from build123d import *

# Parameters (mm, degrees)
SKETCH1_W           = 20
SKETCH1_H           = 46
SKETCH1_R           = 1.25
SKETCH1_R_2         = 4
SKETCH1_R_3         = 1.5
BOSS_EXTRUDE1_DEPTH = 3
SKETCH2_W           = 20
SKETCH2_H           = 13.653393661
CUT_EXTRUDE4_DEPTH  = 26.258661881


with BuildPart() as part:
    # Sketch1 → Boss-Extrude1 (new body)
    with BuildSketch(Plane(origin=(0, 0, 0), x_dir=(1, 0, 0), z_dir=(0, 1, 0))):
        Rectangle(SKETCH1_W, SKETCH1_H)
        with Locations(Location((0, 18, 0), (0, 0, 270))):
            Circle(SKETCH1_R, mode=Mode.SUBTRACT)
        with Locations(Location((0, 1, 0), (0, 0, 270))):
            Circle(SKETCH1_R, mode=Mode.SUBTRACT)
        with Locations(Location((0, 9.5, 0), (0, 0, 270))):
            Circle(SKETCH1_R_2, mode=Mode.SUBTRACT)
        with Locations(Location((0, -13, 0), (0, 0, 270))):
            Circle(SKETCH1_R_3, mode=Mode.SUBTRACT)
    extrude(amount=BOSS_EXTRUDE1_DEPTH)

    # Sketch2 → Cut-Extrude4 (cut, through all)
    with BuildSketch(Plane(origin=(0, 3, 0), x_dir=(1, 0, 0), z_dir=(0, 1, 0))):
        with Locations((0, -29.826696831)):
            Rectangle(SKETCH2_W, SKETCH2_H)
        with BuildLine():
            Line((10, -23), (10, -16.653393661))
            ThreePointArc((10, -16.653393661), (0, -18.5), (-10, -16.653393661))
            Line((-10, -16.653393661), (-10, -23))
            Line((-10, -23), (10, -23))
        make_face()
    extrude(amount=-CUT_EXTRUDE4_DEPTH, mode=Mode.SUBTRACT)


solid = part.part
CAD build for the part. Positions are in the model's coordinates, mm. Coordinates: 2 decimals unless noted, no trailing zeros. Order: outer loops, then holes, each group sorted by start corner. A loop starts at its lowest first (then second) coordinate and runs counter-clockwise, first axis right, second up.
Item 1: Pin check, flat tips, straight feed: pin 1 Ø5 at (x, z) = (-7.5, 8.5) entering from -Y; pin 2 Ø1.5 at (x, y) = (-2.5, 1) entering from +Z. Stop position of each tip, or through.
Check sheet entries:
pin 1: stops at y = 0
pin 2: stops at z = 18.45
Item 2: Band-saw the part on B-B on x = 0. List the corners of the cut face in (y, z).
Check sheet entries:
outline: (0, -23) - (3, -23) - (3, -19.25) - (0, -19.25) - close; (0, -16.75) - (3, -16.75) - (3, -13.5) - (0, -13.5) - close; (0, -5.5) - (3, -5.5) - (3, -2.25) - (0, -2.25) - close; (0, 0.25) - (3, 0.25) - (3, 11.5) - (0, 11.5) - close; (0, 14.5) - (3, 14.5) - (3, 18.5) - (0, 18.5) - close
Item 3: Band-saw the part on C-C on y = 2.5. List the corners of the cut face in (x, z).
Check sheet entries:
outline: (-10, -23) - (10, -23) - (10, 16.65) arc R28 ccw to (-10, 16.65) - close; hole circle Ø8 at (0, -9.5); hole circle Ø3 at (0, 13); hole circle Ø2.5 at (0, -18); hole circle Ø2.5 at (0, -1)
Item 4: Band-saw the part on D-D on z = 13. List the corners of the cut face in (x, y), plus the area to 3 significant figures.
Check sheet entries:
outline: (-10, 0) - (-1.5, 0) - (-1.5, 3) - (-10, 3) - close; (1.5, 0) - (10, 0) - (10, 3) - (1.5, 3) - close
area: 51.0 mm2
Item 5: Two-plate mould, pull along Z, no slides. Class faces 1 (the face through (-2.4, 1.5, -12.7)), 2 (the face through (-10, 1, -3)), 3 (the face through (0.1, 1.5, 18.5)), 4 (the face through (0.07, 1.48, 11.5)): +Z half, -Z half, draft (parallel to the pull), parting line (faces both ways), or undercut.
Check sheet entries:
face 1: undercut
face 2: draft
face 3: +Z half
face 4: undercut
Item 6: Band-saw the part on A-A on z = -1. List the corners of the cut face in (x, y).
Check sheet entries:
outline: (-10, 0) - (-1.25, 0) - (-1.25, 3) - (-10, 3) - close; (1.25, 0) - (10, 0) - (10, 3) - (1.25, 3) - close
Item 7: Drill centre lines: L1, parallel to Z at x = 0.75, y = 2.6; L2, parallel to X at y = 1.25, z = 13; L3, parallel to Z at x = 0.25, y = 1. Where is each one in solid material? Low to high.
Check sheet entries:
L1: z = -23 to -19, -17 to -13.43, -5.57 to -2, 0 to 11.7, 14.3 to 18.49
L2: x = -10 to -1.5, 1.5 to 10
L3: z = -23 to -19.22, -16.78 to -13.49, -5.51 to -2.22, 0.22 to 11.52, 14.48 to 18.5
